The model under review builds one solid part; all positions refer to its coordinate system, in mm. Face numbers are marked on the shaded views. A direction names the side the tool comes from. Give positions to 0.01 mm unless a question says otherwise; leave off trailing zeros. Loops run counter-clockwise (first coordinate to the right, second up) from the corner with the lowest first, then second, coordinate; pieces in that order, holes last. Notation, with made-up numbers: M -29.5,11.25 L -7.5,11.25 A28 ccw -7.5,40.25 Z; hole C 29.5,79.25 d5. An arc over 180 degrees is marked long. Return JSON: item names as keys, results as strings.
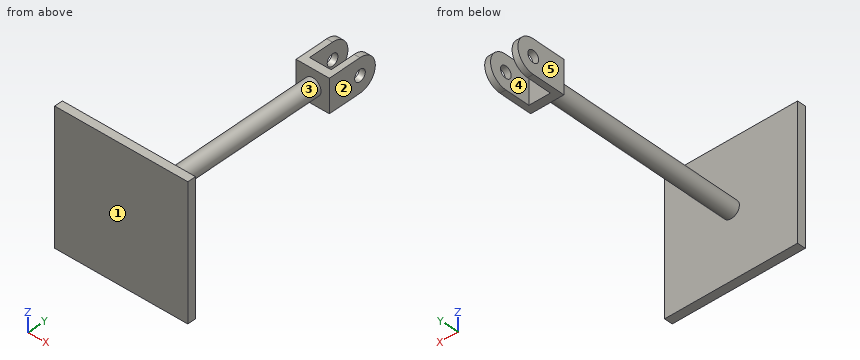
```python
from build123d import *

# Parameters (mm, degrees)
ESBO_O10_W               = 80
ESBO_O10_H               = 80
RESSALTO_EXTRUS_O4_DEPTH = 5
ESBO_O11_R               = 5
RESSALTO_EXTRUS_O5_DEPTH = 120
ESBO_O12_W               = 20
ESBO_O12_H               = 20
RESSALTO_EXTRUS_O6_DEPTH = 5
ESBO_O13_R               = 3.5
RESSALTO_EXTRUS_O7_DEPTH = 10
ESBO_O16_W               = 12.944950436
ESBO_O16_H               = 50
CORTE_EXTRUS_O8_DEPTH    = 20


with BuildPart() as part:
    # Esboço10 → Ressalto-extrusão4 (new body)
    with BuildSketch(Plane(origin=(0, 0, 0), x_dir=(1, 0, 0), z_dir=(0, 1, 0))):
        Rectangle(ESBO_O10_W, ESBO_O10_H)
    extrude(amount=RESSALTO_EXTRUS_O4_DEPTH)

    # Esboço11 → Ressalto-extrusão5 (add)
    with BuildSketch(Plane(origin=(0, 5, 0), x_dir=(1, 0, 0), z_dir=(0, 1, 0))):
        with Locations(Location((0, 0, 0), (0, 0, 270))):
            Circle(ESBO_O11_R)
    extrude(amount=RESSALTO_EXTRUS_O5_DEPTH)

    # Esboço12 → Ressalto-extrusão6 (add)
    with BuildSketch(Plane(origin=(0, 125, 0), x_dir=(1, 0, 0), z_dir=(0, 1, 0))):
        Rectangle(ESBO_O12_W, ESBO_O12_H)
    extrude(amount=RESSALTO_EXTRUS_O6_DEPTH)

    # Esboço13 → Ressalto-extrusão7 (add, symmetric)
    with BuildSketch(Plane(origin=(0, 0, 0), x_dir=(0, 0, -1), z_dir=(1, 0, 0))):
        with BuildLine():
            Line((10, 130), (-10, 130))
            Line((-10, 130), (-10, 145))
            ThreePointArc((-10, 145), (0, 155), (10, 145))
            Line((10, 145), (10, 130))
        make_face()
        with Locations((0, 145)):
            Circle(ESBO_O13_R, mode=Mode.SUBTRACT)
    extrude(amount=RESSALTO_EXTRUS_O7_DEPTH, both=True)

    # Esboço16 → Corte-extrusão8 (cut, symmetric)
    with BuildSketch(Plane.XY):
        with Locations((0, 155)):
            Rectangle(ESBO_O16_W, ESBO_O16_H)
    extrude(amount=CORTE_EXTRUS_O8_DEPTH, both=True, mode=Mode.SUBTRACT)


solid = part.part
```
1) The part is to be moulded in two halves that separate along Y. For the marked faces 1, 2 and 3, say which applies: released by +Y, released by -Y, zero draft, split by the parting line, or undercut.
From the geometry:
{"face 1": "released by -Y", "face 2": "zero draft", "face 3": "undercut"}
2) Consider section B-B on y = 134. Write out the cut boundary in (x, z).
From the geometry:
{"outline": "M -10,-10 L -6.47,-10 L -6.47,10 L -10,10 Z; M 6.47,-10 L 10,-10 L 10,10 L 6.47,10 Z"}
3) Consider section C-C on x = 0. Write out the cut boundary in (y, z), then the cut area to 3 significant figures.
From the geometry:
{"outline": "M 0,-40 L 5,-40 L 5,-5 L 125,-5 L 125,-10 L 130,-10 L 130,10 L 125,10 L 125,5 L 5,5 L 5,40 L 0,40 Z", "area": "1,700 mm²"}
4) Tool access review of the marked faces 4 and 5: name each direction out of +Z, -Z, +X, -X, +Y, -Y from which nothing blocks a thin tool from reaching the whole face with its end or side.
From the geometry:
{"face 4": "+Z, -Z, +Y", "face 5": "+Z, -Z, -X, +Y"}
5) Wall thickness on L1, parallel to Y at x = 7, z = 0; L2, parallel to Z at x = 8, y = 145; L3, parallel to Y at x = 9.5, z = 1.5: over which ranges is each line inside the solid? List them lowest first. Write a range as from..to.
From the geometry:
{"L1": "0..5, 125..141.5, 148.5..155", "L2": "-10..-3.5, 3.5..10", "L3": "0..5, 125..141.84, 148.16..154.89"}
6) Insertion check: pin 1 (6 mm diameter, centred on x = -22.5, z = -13.5, fed in from +Y); pin 2 (5 mm diameter, centred on x = 31, z = 18.5, fed in from -Y); pin 3 (10 mm diameter, centred on y = 121, z = -11, fed in from -X); pin 4 (1 mm diameter, centred on y = 84.5, z = 5, fed in from +X). Each pin has a flat end and moves straight along its axis. Give the tip position at first contact, or say it passes through.
From the geometry:
{"pin 1": "y = 5", "pin 2": "y = 0", "pin 3": "x = -10", "pin 4": "x = 2.18"}
7) Consider section A-A on z = 0. Write out the cut boundary in (x, y).
From the geometry:
{"outline": "M -40,0 L 40,0 L 40,5 L 5,5 L 5,125 L 10,125 L 10,141.5 L 6.47,141.5 L 6.47,130 L -6.47,130 L -6.47,141.5 L -10,141.5 L -10,125 L -5,125 L -5,5 L -40,5 Z; M -10,148.5 L -6.47,148.5 L -6.47,155 L -10,155 Z; M 6.47,148.5 L 10,148.5 L 10,155 L 6.47,155 Z"}
8) Consider section D-D on y = 77. Write out the cut boundary in (x, z).
From the geometry:
{"outline": "C 0,0 d10"}
